Geometry: final body of the model. Coordinates: model frame, mm. Face numbers are marked on the shaded views. Coordinates: 2 decimals unless noted, no trailing zeros. Loops run counter-clockwise (first coordinate to the right, second up) from the corner with the lowest first, then second, coordinate; pieces in that order, holes last. Notation, with made-up numbers: (-27.75, -39.5) - (19.25, -39.5) arc R21 cw to (19.25, -19.5) - close; hole circle Ø4 at (65, 2.25). An arc over 180 degrees is marked (long way). Answer in a Markdown table with one row per item.
from build123d import *

# Parameters (mm, degrees)
SKETCH1_R           = 3.5
SKETCH1_R_2         = 2
BOSS_EXTRUDE1_DEPTH = 5
SKETCH2_R           = 2
SKETCH2_R_2         = 0.7
BOSS_EXTRUDE2_DEPTH = 2


with BuildPart() as part:
    # Sketch1 → Boss-Extrude1 (new body)
    with BuildSketch(Plane.XY):
        Circle(SKETCH1_R)
        Circle(SKETCH1_R_2, mode=Mode.SUBTRACT)
    extrude(amount=BOSS_EXTRUDE1_DEPTH)

    # Sketch2 → Boss-Extrude2 (add)
    with BuildSketch(Plane(origin=(0, 0, 0), x_dir=(-1, 0, 0), z_dir=(0, 0, -1))):
        with BuildLine():
            Line((0.499445817, 3.464181559), (13, 2.5))
            ThreePointArc((13, 2.5), (15.5, 0), (13, -2.5))
            Line((13, -2.5), (0.499445817, -3.464181559))
            ThreePointArc((0.499445817, -3.464181559), (-3.5, 0), (0.499445817, 3.464181559))
        make_face()
        with Locations(Location((0, 0, 0), (0, 0, 180))):
            Circle(SKETCH2_R, mode=Mode.SUBTRACT)
        with Locations((7, 0)):
            Circle(SKETCH2_R_2, mode=Mode.SUBTRACT)
        with Locations((10, 0)):
            Circle(SKETCH2_R_2, mode=Mode.SUBTRACT)
        with Locations((13, 0)):
            Circle(SKETCH2_R_2, mode=Mode.SUBTRACT)
    extrude(amount=-BOSS_EXTRUDE2_DEPTH)


solid = part.part
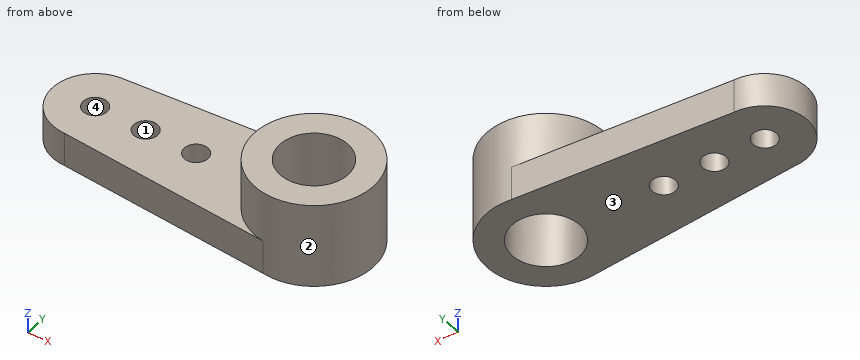
(1) Cut plane A-A on y = 0. Output: boundary loops of the cut face in (x, z), then the cut area to 3 significant figures.
Verdict:
| item | result |
|---|---|
| outline | (-15.5, 0) - (-13.7, 0) - (-13.7, 2) - (-15.5, 2) - close; (-12.3, 0) - (-10.7, 0) - (-10.7, 2) - (-12.3, 2) - close; (-9.3, 0) - (-7.7, 0) - (-7.7, 2) - (-9.3, 2) - close; (-6.3, 0) - (-2, 0) - (-2, 5) - (-3.5, 5) - (-3.5, 2) - (-6.3, 2) - close; (2, 0) - (3.5, 0) - (3.5, 5) - (2, 5) - close |
| area | 30.6 mm² |
(2) Cut plane C-C on z = 0.3. Output: boundary loops of the cut face in (x, y).
Verdict:
| item | result |
|---|---|
| outline | (-13, -2.5) - (-0.5, -3.46) arc R3.5 ccw (long way) to (-0.5, 3.46) - (-13, 2.5) arc R2.5 ccw to start; hole circle Ø1.4 at (-13, 0); hole circle Ø1.4 at (-10, 0); hole circle Ø1.4 at (-7, 0); hole circle Ø4 at (0, 0) |
(3) Cut plane D-D on y = -1.5. Output: boundary loops of the cut face in (x, z).
Verdict:
| item | result |
|---|---|
| outline | (-15, 0) - (-1.32, 0) - (-1.32, 5) - (-3.16, 5) - (-3.16, 2) - (-15, 2) - close; (1.32, 0) - (3.16, 0) - (3.16, 5) - (1.32, 5) - close |
(4) Ray query, probe 1 along Y at (x, z) = (-13, 1.15); probe 2 along Y at (x, z) = (0, 3.6); probe 3 along Z at (x, y) = (-11.5, 0.5). Return the intervals inside material, ascending.
Verdict:
| item | result |
|---|---|
| probe 1 | y = -2.5 to -0.7, 0.7 to 2.5 |
| probe 2 | y = -3.5 to -2, 2 to 3.5 |
| probe 3 | z = 0 to 2 |
(5) Cut plane B-B on x = 0. Output: boundary loops of the cut face in (y, z).
Verdict:
| item | result |
|---|---|
| outline | (-3.5, 0) - (-2, 0) - (-2, 5) - (-3.5, 5) - close; (2, 0) - (3.5, 0) - (3.5, 5) - (2, 5) - close |
(6) Pull-direction query (Y, two-part tool) for the marked faces 1, 2, 3 and 4; classes: pulls with the +Y half, pulls with the -Y half, needs draft (parallel to the pull), parting line crosses it, or undercut.
Verdict:
| item | result |
|---|---|
| face 1 | undercut |
| face 2 | parting line crosses it |
| face 3 | needs draft |
| face 4 | undercut |
(7) First-contact query: pin 1 Ø3 at (y, z) = (-2.5, 2.5) entering from +X; pin 2 Ø1.5 at (y, z) = (-2, 1.5) entering from +X; pin 3 Ø1.8 at (x, y) = (-7, 0) entering from +Z; pin 4 Ø2 at (x, z) = (-7, 3.5) entering from -Y. Flat tips, straight axial feed; report the tip coordinate or a pass-through.
Verdict:
| item | result |
|---|---|
| pin 1 | stops at x = 3.35 |
| pin 2 | stops at x = 3.27 |
| pin 3 | stops at z = 2 |
| pin 4 | passes through |
